Can you work these out from the model? Positions are in its coordinate system, mm. A direction names the side the tool comes from. Round coordinates to 2 decimals unless told otherwise and drop trailing zeros. Loops run counter-clockwise (first coordinate to the right, second up) from the corner with the lowest first, then second, coordinate; pieces in that order, holes last.
from build123d import *

# Parameters (mm, degrees)
F0_R     = 27.5
F0_R_2   = 7.5
F1_DEPTH = 1
F3_DEPTH = 15
F4_COUNT = 6
F5_DEPTH = 16


with BuildPart() as f1:
    # F0 (on Top) → F1 (new body)
    with BuildSketch(Plane.XY):
        Circle(F0_R)
        Circle(F0_R_2, mode=Mode.SUBTRACT)
        Circle(F0_R_2)
        Polygon((-3.25, 1.876388), (0, 3.752777), (3.25, 1.876388), (3.25, -1.876388), (0, -3.752777), (-3.25, -1.876388), align=None, mode=Mode.SUBTRACT)
    extrude(amount=F1_DEPTH)

    # F2 (on face) → F3 (join)
    with BuildSketch(Plane.XY.offset(1)):
        with BuildLine():
            ThreePointArc((-27.43591, 1.876388), (-27.5, 0), (-27.43591, -1.876388))
            ThreePointArc((-27.43591, -1.876388), (-15.342955, -3.824912), (-3.25, -1.876388))
            Line((-3.25, -1.876388), (-3.25, 1.876388))
            ThreePointArc((-3.25, 1.876388), (-15.342955, -0.072135), (-27.43591, 1.876388))
        make_face()
        with BuildLine():
            ThreePointArc((3.25, -1.876388), (15.342955, 0.072135), (27.43591, -1.876388))
            ThreePointArc((27.43591, -1.876388), (27.483973, -0.938741), (27.5, 0))
            ThreePointArc((27.5, 0), (27.483973, 0.938741), (27.43591, 1.876388))
            ThreePointArc((27.43591, 1.876388), (15.342955, 3.824912), (3.25, 1.876388))
            Line((3.25, 1.876388), (3.25, -1.876388))
        make_face()
    extrude(amount=F3_DEPTH)



with BuildPart() as f4_1:
    # F4: instance of F1
    add(f1.part.rotate(Axis((0, 0, 0), (0, 0, 1)), 1 * 360 / F4_COUNT))


with BuildPart() as f4_2:
    # F4: instance of F1
    add(f1.part.rotate(Axis((0, 0, 0), (0, 0, 1)), 2 * 360 / F4_COUNT))


with BuildPart() as f4_3:
    # F4: instance of F1
    add(f1.part.rotate(Axis((0, 0, 0), (0, 0, 1)), 3 * 360 / F4_COUNT))


with BuildPart() as f4_4:
    # F4: instance of F1
    add(f1.part.rotate(Axis((0, 0, 0), (0, 0, 1)), 4 * 360 / F4_COUNT))


with BuildPart() as f4_5:
    # F4: instance of F1
    add(f1.part.rotate(Axis((0, 0, 0), (0, 0, 1)), 5 * 360 / F4_COUNT))


with BuildPart() as f1_1:
    add(f1.part)

    add(f4_1.part)  # F5 merges F4_1

    add(f4_2.part)  # F5 merges F4_2

    add(f4_3.part)  # F5 merges F4_3

    add(f4_4.part)  # F5 merges F4_4

    add(f4_5.part)  # F5 merges F4_5
    # F0 (on Top) → F5 (join)
    with BuildSketch(Plane.XY):
        Circle(F0_R_2)
        Polygon((-3.25, 1.876388), (0, 3.752777), (3.25, 1.876388), (3.25, -1.876388), (0, -3.752777), (-3.25, -1.876388), align=None, mode=Mode.SUBTRACT)
    extrude(amount=F5_DEPTH)


solid = f1_1.part
(1) Will these pins go through, and if not, where does the flat tip stop? P1, Ø1.5, axis at x = -12, y = -5, coming from the +Z side; P2, Ø2, axis at y = -22, z = 8.5, coming from the +X side; P3, Ø4, axis at x = -20.5, z = 11, coming from the +Y side.
Worked answers:
P1: stops at z = 1
P2: stops at x = 15.34
P3: stops at y = 0.6
(2) If we section it at B-B, the plane y = -11: List the corners of the cut face in (x, z) for me, then the cut area to 3 significant figures.
Worked answers:
outline: (-25.2, 0) - (25.2, 0) - (25.2, 1) - (10.76, 1) - (10.76, 16) - (6.33, 16) - (6.33, 1) - (-2.26, 1) - (-2.26, 16) - (-6.37, 16) - (-6.37, 1) - (-25.2, 1) - close
area: 179 mm2
(3) If we mould it in two halves opening along X, with no side actions, what happens to faces 1 (the cylindrical face through (-5.961, -26.846, 0.493)), 2 (the cylindrical face through (-5.4, -16.9, 8.4)), 3 (the cylindrical face through (-11.961, 13.177, 8.395))? For each: released by +X, released by -X, zero draft, split by the parting line, or undercut.
Worked answers:
face 1: split by the parting line
face 2: undercut
face 3: released by -X
(4) If we section it at C-C, the plane x = 13: List the corners of the cut face in (y, z) for me, then the cut area to 3 significant figures.
Worked answers:
outline: (-24.23, 0) - (24.23, 0) - (24.23, 16) - (20.55, 16) - (20.55, 1) - (3.75, 1) - (3.75, 16) - (0, 16) - (0, 1) - (-15.39, 1) - (-15.39, 16) - (-24.23, 16) - close
area: 293 mm2
(5) For faces 4 (the cylindrical face through (-8.7, -15.1, 8.4)), 5 (the flat face through (1.65, -2.8, 7.89)), 6 (the cylindrical face through (17.38, 0.02, 8.4)), which set-ups out of +Z, -Z, +X, -X, +Y, -Y let a thin tool reach every point of the face, with its end or its side?
Worked answers:
face 4: +Z, -X
face 5: +Z, -Z
face 6: +Z
(6) If we section it at D-D, the plane y = 12.5: List the corners of the cut face in (x, z) for me.
Worked answers:
outline: (-24.49, 0) - (24.49, 0) - (24.49, 1) - (7.15, 1) - (7.15, 16) - (2.94, 16) - (2.94, 1) - (-7.29, 1) - (-7.29, 16) - (-11.61, 16) - (-11.61, 1) - (-24.49, 1) - close
(7) If I drill on line 1 (Y direction, x = -8, z = 14.75); line 2 (Y direction, x = 6.5, z = 13.5); line 3 (Z direction, x = -23.5, y = -8), over which ranges is the centre line in solid material (lowest first)?
Worked answers:
line 1: y = -20.45 to -13.99, -3.12 to 0.63, 6.95 to 13.72
line 2: y = -11.26 to -5.14, -3.74 to 3.74, 11.26 to 18.51
line 3: z = 0 to 1
